from build123d import *

# Parameters (mm, degrees)
SKETCH1_R           = 12.5
BOSS_EXTRUDE1_DEPTH = 2
SKETCH2_R           = 8.5
CUT_EXTRUDE1_DEPTH  = 2
SKETCH5_W           = 2
SKETCH5_H           = 1.2
BOSS_EXTRUDE3_DEPTH = 17
SKETCH8_R           = 0.5
BOSS_EXTRUDE4_DEPTH = 4.8
BOSS_EXTRUDE5_START = 4
SKETCH9_R           = 0.5
BOSS_EXTRUDE5_DEPTH = 4


with BuildPart() as part:
    # Sketch1 → Boss-Extrude1 (new body)
    with BuildSketch(Plane.XY):
        Circle(SKETCH1_R)
    extrude(amount=BOSS_EXTRUDE1_DEPTH)

    # Sketch2 → Cut-Extrude1 (cut)
    with BuildSketch(Plane.XY.offset(2)):
        Circle(SKETCH2_R)
    extrude(amount=-CUT_EXTRUDE1_DEPTH, mode=Mode.SUBTRACT)

    # Sketch5 → Boss-Extrude3 (add)
    with BuildSketch(Plane(origin=(0, 0, 0), x_dir=(-1, 0, 0), z_dir=(0, 0, -1))):
        with Locations((0, -10)):
            Rectangle(SKETCH5_W, SKETCH5_H)
        with Locations((0, 10)):
            Rectangle(SKETCH5_W, SKETCH5_H)
    extrude(amount=BOSS_EXTRUDE3_DEPTH)

    # Sketch8 → Boss-Extrude4 (add)
    with BuildSketch(Plane(origin=(0, 10.6, 0), x_dir=(1, 0, 0), z_dir=(0, 1, 0))):
        with Locations(Location((0, 2, 0), (0, 0, 90))):
            Circle(SKETCH8_R)
        with Locations(Location((0, 15, 0), (0, 0, 90))):
            Circle(SKETCH8_R)
    extrude(amount=BOSS_EXTRUDE4_DEPTH)

    # Sketch9 → Boss-Extrude5 (add)
    with BuildSketch(Plane.XZ.offset(10.6).offset(BOSS_EXTRUDE5_START)):
        with Locations(Location((0, -2, 0), (0, 0, 270))):
            Circle(SKETCH9_R)
        with Locations(Location((0, -15, 0), (0, 0, 270))):
            Circle(SKETCH9_R)
    extrude(amount=-BOSS_EXTRUDE5_DEPTH)


solid = part.part
Can you work these out from the model? Positions are in its coordinate system, mm. A direction names the side the tool comes from. Give positions to 0.01 mm unless a question says otherwise; leave off trailing zeros. Loops run counter-clockwise (first coordinate to the right, second up) from the corner with the lowest first, then second, coordinate; pieces in that order, holes last. Notation, with made-up numbers: (52, 76) - (89, 76) arc R33 ccw to (89, 109) - close; hole circle Ø11 at (35.5, -21.5). An arc over 180 degrees is marked (long way). Answer as a JSON object with one key per item and string values.
Q1. If I drill on L1, parallel to Y at x = 0, z = 0.65; L2, parallel to Z at x = -0.25, y = -12; L3, parallel to Z at x = 2.25, y = -10, over which ranges is the centre line in solid material (lowest first)?
Geometry says:
{"L1": "-12.5 to -8.5, 8.5 to 12.5", "L2": "-15.43 to -14.57, -2.43 to -1.57, 0 to 2", "L3": "0 to 2"}
Q2. Will these pins go through, and if not, where does the flat tip stop? P1, Ø12, axis at x = 1.5, y = 1.5, coming from the -Z side; P2, Ø1.3, axis at y = -10, z = -6.5, coming from the -X side; P3, Ø1, axis at y = 10, z = -9.5, coming from the +X side; P4, Ø0.6, axis at x = 0, z = -9.5, coming from the +Y side.
Geometry says:
{"P1": "through", "P2": "x = -1", "P3": "x = 1", "P4": "y = 10.6"}
Q3. Which directions (+Z, -Z, +X, -X, +Y, -Y) give clear straight access to the entire face, cutting with the end or side of a thin tool? Please do faces 1 (the flat face through (-1, 10, -8)), 2 (the cylindrical face through (0, -12.6, -1.5)), 3 (the flat face through (0, 9.4, -8)), 4 (the flat face through (1, -10, -8)).
Geometry says:
{"face 1": "-Z, -X, +Y, -Y", "face 2": "-Y", "face 3": "-Z, +X, -X", "face 4": "-Z, +X, +Y, -Y"}
Q4. Imagine slicing it at C-C on z = -2. Write out the boundary of the cut face in (x, y), plus the area to 3 significant figures.
Geometry says:
{"outline": "(-1, -10.6) - (-0.5, -10.6) - (-0.5, -14.6) - (0.5, -14.6) - (0.5, -10.6) - (1, -10.6) - (1, -9.4) - (-1, -9.4) - close; (-1, 9.4) - (1, 9.4) - (1, 10.6) - (0.5, 10.6) - (0.5, 15.4) - (-0.5, 15.4) - (-0.5, 10.6) - (-1, 10.6) - close", "area": "13.6 mm²"}
Q5. Imagine slicing it at B-B on y = 0. Write out the boundary of the cut face in (x, z).
Geometry says:
{"outline": "(-12.5, 0) - (-8.5, 0) - (-8.5, 2) - (-12.5, 2) - close; (8.5, 0) - (12.5, 0) - (12.5, 2) - (8.5, 2) - close"}
Q6. If we mould it in two halves opening along Z, with no side actions, what happens to faces 5 (the flat face through (0, -14.6, -2)), 6 (the flat face through (0, -10, -17)), 7 (the cylindrical face through (0, 13, -1.5)), 8 (the flat face through (0, -10.6, -8))? For each: pulls with the +Z half, pulls with the -Z half, needs draft (parallel to the pull), parting line crosses it, or undercut.
Geometry says:
{"face 5": "needs draft", "face 6": "pulls with the -Z half", "face 7": "undercut", "face 8": "undercut"}
Q7. Imagine slicing it at D-D on y = -6.75. Write out the boundary of the cut face in (x, z).
Geometry says:
{"outline": "(-10.52, 0) - (-5.17, 0) - (-5.17, 2) - (-10.52, 2) - close; (5.17, 0) - (10.52, 0) - (10.52, 2) - (5.17, 2) - close"}
